Autodesk Inventor part; units mm, degrees
ref_plane "Work Plane1" through (0, 10, 0) normal (0, 1, 0) x (1, 0, 0)
ref_plane "YZ Plane" through (0, 0, 0) normal (1, 0, 0) x (0, 1, 0)
ref_plane "XZ Plane" through (0, 0, 0) normal (0, 1, 0) x (-1, 0, 0)
sketch "Sketch1" plane through (0, 0, 0) normal (0, 1, 0) x (-1, 0, 0)
  circle A0 centre (0, 0) radius 1.5
  dimension "d0" = 3
extrude "Extrusion1" add sketch "Sketch1" along normal blind 8
thread "Thread1"
ref_plane "Work Plane1" through (0, 10, 0) normal (0, 1, 0) x (1, 0, 0)
sketch "Sketch4" plane through (0, 10, 0) normal (0, 1, 0) x (1, 0, 0)
  circle A0 centre (0, 0) radius 2.5
  dimension "d14" = 5
loft "Loft1" add profiles "Sketch4" section 2 edges at (1.5, 8, 0)
sketch "Sketch5" plane through (0, 10, 0) normal (0, 1, 0) x (1, 0, 0)
  circle A0 centre (0, 0) radius 2.5
  line L0 (-2.4495, 0.5) -> (2.4495, 0.5)
  line L1 (-2.4495, -0.5) -> (2.4495, -0.5)
  line L2 (0, 0) -> (2.0973, 0) construction
  dimension "d19" = 1
extrude "Extrusion4" cut sketch "Sketch5" against normal blind 1 contours A0 L1 L0
properties part number "Screw_CountersunkHead_3x10" material "Steel, Galvanized"
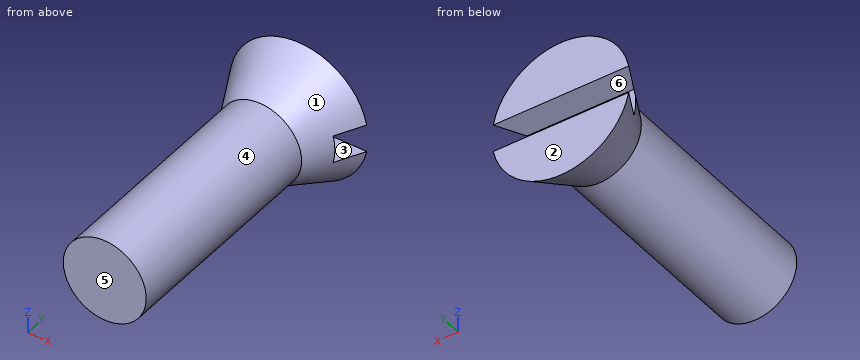
Source: CAD feature listing. Evaluate the final solid. Frame: model axes, mm. Face numbers are marked on the shaded views. A direction names the side the tool comes from. Coordinates: 2 decimals unless noted, no trailing zeros. Loops run counter-clockwise (first coordinate to the right, second up) from the corner with the lowest first, then second, coordinate; pieces in that order, holes last. Notation, with made-up numbers: (25, -20) - (43, -20) arc R27 ccw to (43, 13) - close; hole circle Ø10 at (14.5, 41). An arc over 180 degrees is marked (long way). One line per item, written item: value. Start each with the question number.
1. Set-up query: the marked faces 4, 5 and 6. Return all of +Z, -Z, +X, -X, +Y, -Y with unobstructed straight access to the full face (end or side cutting, diameter ignored); none if empty.
2. Ray query, L1, parallel to X at y = 8.5, z = 0.9; L2, parallel to Y at x = -1.2, z = 0.4; L3, parallel to Y at x = 1.85, z = 0.75. Return the intervals inside material, ascending.
3. Section B-B (y = 8.5). Return the cut outline in (x, z), and give its area (3 significant figures).
4. Mould query, pull axis Z, two halves, no side actions, for the marked faces 1, 2 and 3. Classes: pulls with the +Z half, pulls with the -Z half, needs draft (parallel to the pull), parting line crosses it, or undercut.
5. Section C-C (y = 1.75). Return the cut outline in (x, z), and give its area (3 significant figures).
6. Section A-A (x = 0). Return the cut outline in (y, z), and give its area (3 significant figures).
7. Contact query for a flat-ended pin moving along its axis: P1, Ø0.5, axis at x = -1, y = 9.5, coming from the +Z side. Output: stop coordinate, or through.
Verdict:
1. face 4: -Y
1. face 5: +Z, -Z, +X, -X, -Y
1. face 6: +X, -X, +Y
2. L1: x = -1.5 to 1.5
2. L2: y = 0 to 9
2. L3: y = 8.99 to 10
3. outline: circle Ø3.5 at (0, 0)
3. area: 9.62 mm2
4. face 1: parting line crosses it
4. face 2: needs draft
4. face 3: undercut
5. outline: circle Ø3 at (0, 0)
5. area: 7.07 mm2
6. outline: (0, -1.5) - (8, -1.5) - (10, -2.5) - (10, -0.5) - (9, -0.5) - (9, 0.5) - (10, 0.5) - (10, 2.5) - (8, 1.5) - (0, 1.5) - close
6. area: 31.0 mm2
7. P1: stops at z = 2.19
